Geometry: see drawing. Coordinates: mm, zero at the bounding-box minimum. A direction names the side the tool comes from. Coordinates: 2 decimals unless noted, no trailing zeros. Order: outer loops, then holes, each group sorted by start corner. A loop starts at its lowest first (then second) coordinate and runs counter-clockwise, first axis right, second up.
Item 1: Section A-A on y = 32.5. Return the cut outline in (x, z), then the cut area to 3 significant figures.
Item 2: Section C-C on z = 37. Return the cut outline in (x, y), then the cut area to 3 significant figures.
Item 3: Section B-B on x = 5. Return the cut outline in (y, z), then the cut area to 3 significant figures.
Item 4: Contact query for flat-ended pins moving along their axis: P1, Ø6, axis at y = 32.5, z = 31, coming from the +X side; P2, Ø5, axis at x = 60, y = 32.5, coming from the +Z side; P3, Ø4, axis at y = 26.5, z = 35, coming from the +X side. Output: stop coordinate, or through.
Item 5: Reachability of the marked faces 1 and 2 from +Z, -Z, +X, -X, +Y, -Y: full face, straight path, thin tool, end or side. Return the list, or none.
Item 6: Ray query, line 1 (Y direction, x = 32.5, z = 1.95); line 2 (Y direction, x = 32, z = 1); line 3 (Z direction, x = 10.5, y = 14). Return the intervals inside material, ascending.
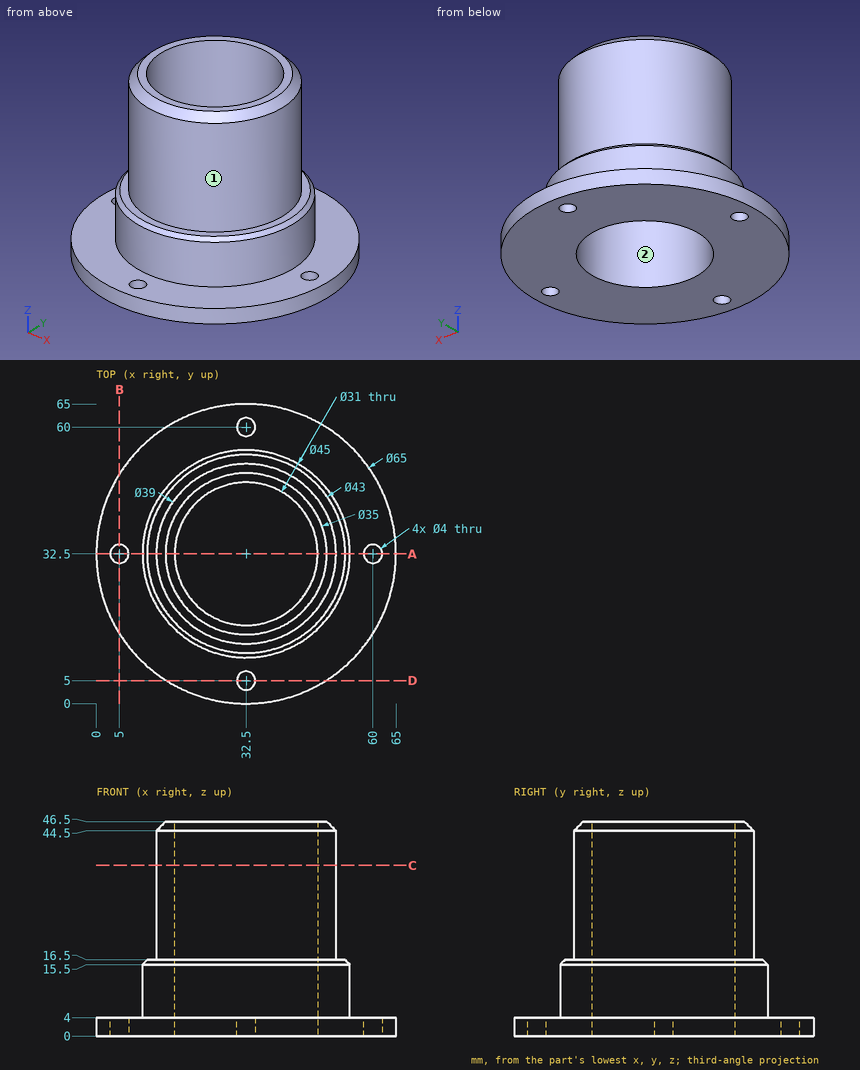
Answer list:
1. outline: (0, 0) - (3, 0) - (3, 4) - (0, 4) - close; (7, 0) - (17, 0) - (17, 46.5) - (15, 46.5) - (13, 44.5) - (13, 16.5) - (11, 16.5) - (10, 15.5) - (10, 4) - (7, 4) - close; (48, 0) - (58, 0) - (58, 4) - (55, 4) - (55, 15.5) - (54, 16.5) - (52, 16.5) - (52, 44.5) - (50, 46.5) - (48, 46.5) - close; (62, 0) - (65, 0) - (65, 4) - (62, 4) - close
1. area: 514 mm2
2. outline: circle Ø39 at (32.5, 32.5); hole circle Ø31 at (32.5, 32.5)
2. area: 440 mm2
3. outline: (15.18, 0) - (30.5, 0) - (30.5, 4) - (15.18, 4) - close; (34.5, 0) - (49.82, 0) - (49.82, 4) - (34.5, 4) - close
3. area: 123 mm2
4. P1: stops at x = 52
4. P2: stops at z = 4
4. P3: stops at x = 51.59
5. face 1: +Z
5. face 2: +Z, -Z
6. line 1: y = 0 to 3, 7 to 17, 48 to 58, 62 to 65
6. line 2: y = 0 to 3.06, 6.94 to 17.01, 47.99 to 58.06, 61.94 to 65
6. line 3: z = 0 to 4
